Check sheet for the modelled part. Datum: model origin and axes. Units: mm. Face numbers are marked on the shaded views. A direction names the side the tool comes from. Round coordinates to 2 decimals unless told otherwise and drop trailing zeros. Loops run counter-clockwise (first coordinate to the right, second up) from the corner with the lowest first, then second, coordinate; pieces in that order, holes last. Notation, with made-up numbers: (-37, 38.5) - (-4, 38.5) arc R36 ccw to (-4, 74.5) - close; hole circle Ø1 at (-18, 37.25). An arc over 180 degrees is marked (long way). Put each result on its own line as item: value. Start each with the question number.
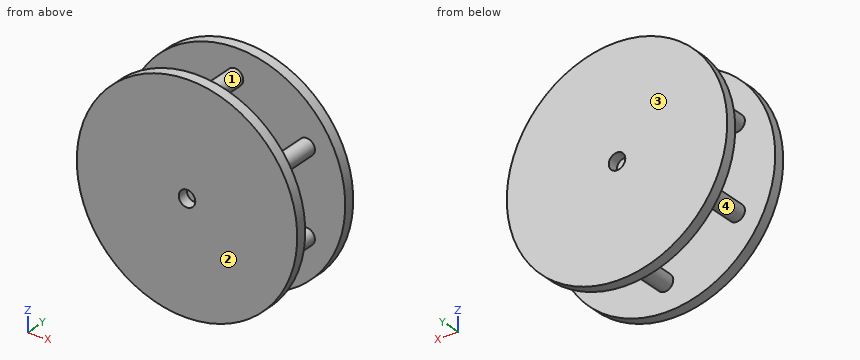
```python
from build123d import *

# Parameters (mm, degrees)
SKETCH1_R           = 50.789558068
BOSS_EXTRUDE1_DEPTH = 5.08
SKETCH3_R           = 3.813733887
BOSS_EXTRUDE2_DEPTH = 25.4
CIRPATTERN1_COUNT   = 6
SKETCH4_R           = 50.789558068
BOSS_EXTRUDE3_DEPTH = 5.08
SKETCH6_R           = 3.81
CUT_EXTRUDE1_DEPTH  = 81.147813554


with BuildPart() as part:
    # Sketch1 → Boss-Extrude1 (new body)
    with BuildSketch(Plane(origin=(0, 0, 0), x_dir=(1, 0, 0), z_dir=(0, 1, 0))):
        with Locations(Location((0, 0, 0), (0, 0, 270))):
            Circle(SKETCH1_R)
    extrude(amount=BOSS_EXTRUDE1_DEPTH)

    # Sketch3 → Boss-Extrude2 (add)
    with BuildSketch(Plane(origin=(0, 5.08, 0), x_dir=(1, 0, 0), z_dir=(0, 1, 0))):
        with Locations(Location((0, 38.1, 0), (0, 0, 270))):
            Circle(SKETCH3_R)
    boss_extrude2 = extrude(amount=BOSS_EXTRUDE2_DEPTH)

    # CirPattern1: Boss-Extrude2 ×6 about axis
    cirpattern1_axis = Axis((0, 0, 0), (0, 1, 0))
    for i in range(1, CIRPATTERN1_COUNT):
        add(boss_extrude2.rotate(cirpattern1_axis, i * 360 / CIRPATTERN1_COUNT))

    # Sketch4 → Boss-Extrude3 (add)
    with BuildSketch(Plane(origin=(0, 30.48, 0), x_dir=(1, 0, 0), z_dir=(0, 1, 0))):
        with Locations(Location((0, 0, 0), (0, 0, 270))):
            Circle(SKETCH4_R)
    extrude(amount=BOSS_EXTRUDE3_DEPTH)

    # Sketch6 → Cut-Extrude1 (cut, through all)
    with BuildSketch(Plane(origin=(0, 35.56, 0), x_dir=(1, 0, 0), z_dir=(0, 1, 0))):
        with Locations(Location((0, 0, 0), (0, 0, 270))):
            Circle(SKETCH6_R)
    extrude(amount=-CUT_EXTRUDE1_DEPTH, mode=Mode.SUBTRACT)


solid = part.part
```
Q1. Depth check by flat-ended pin: pin 1 Ø10 at (y, z) = (13, -27) entering from -X; pin 2 Ø10 at (x, y) = (-3, 25) entering from -Z; pin 3 Ø4 at (x, y) = (-4, 23) entering from +Z; pin 4 Ø1 at (x, y) = (5, 26.5) entering from -Z. Enter the tip coordinate at first touch or a pass-through.
Q2. Cross-section at A-A on x = 0. Enter the section's corners in (y, z).
Q3. Cross-section at C-C on y = 23. Enter the section's corners in (x, z), and give its area (3 significant figures).
Q4. Cross-section at D-D on z = 19.05. Enter the section's corners in (x, y).
Q5. Cross-section at B-B on z = 0. Enter the section's corners in (x, y).
Q6. Draft check along Z on the marked faces 3 and 4. Enter one of: +Z half, -Z half, draft (parallel to the pull), parting line (faces both ways), or undercut.
Q7. Material ranges on line 1 (Y direction, x = -40, z = 2.5); line 2 (X direction, y = 32.45, z = 0); line 3 (Z direction, x = -2.5, y = 19.5), recorded low to high. Write a range as from..to.
Q8. Set-up check for the marked faces 1 and 2: record each of +Z, -Z, +X, -X, +Y, -Y from which the full face is reachable in a straight line by a thin tool's end or side.
Answer list:
1. pin 1: stops at x = -35.41
1. pin 2: stops at z = -41.91
1. pin 3: stops at z = 41.35
1. pin 4: passes through
2. outline: (0, -50.79) - (5.08, -50.79) - (5.08, -41.91) - (30.48, -41.91) - (30.48, -50.79) - (35.56, -50.79) - (35.56, -3.81) - (30.48, -3.81) - (30.48, -34.29) - (5.08, -34.29) - (5.08, -3.81) - (0, -3.81) - close; (0, 3.81) - (5.08, 3.81) - (5.08, 34.29) - (30.48, 34.29) - (30.48, 3.81) - (35.56, 3.81) - (35.56, 50.79) - (30.48, 50.79) - (30.48, 41.91) - (5.08, 41.91) - (5.08, 50.79) - (0, 50.79) - close
3. outline: circle Ø7.63 at (-33, -19.05); circle Ø7.63 at (-33, 19.05); circle Ø7.63 at (0, -38.1); circle Ø7.63 at (0, 38.1); circle Ø7.63 at (33, -19.05); circle Ø7.63 at (33, 19.05)
3. area: 274 mm2
4. outline: (-47.08, 0) - (47.08, 0) - (47.08, 5.08) - (36.81, 5.08) - (36.81, 30.48) - (47.08, 30.48) - (47.08, 35.56) - (-47.08, 35.56) - (-47.08, 30.48) - (-36.81, 30.48) - (-36.81, 5.08) - (-47.08, 5.08) - close; hole (-29.18, 5.08) - (29.18, 5.08) - (29.18, 30.48) - (-29.18, 30.48) - close
5. outline: (-50.79, 0) - (-3.81, 0) - (-3.81, 5.08) - (-50.79, 5.08) - close; (-50.79, 30.48) - (-3.81, 30.48) - (-3.81, 35.56) - (-50.79, 35.56) - close; (3.81, 0) - (50.79, 0) - (50.79, 5.08) - (3.81, 5.08) - close; (3.81, 30.48) - (50.79, 30.48) - (50.79, 35.56) - (3.81, 35.56) - close
6. face 3: draft
6. face 4: undercut
7. line 1: y = 0..5.08, 30.48..35.56
7. line 2: x = -50.79..-3.81, 3.81..50.79
7. line 3: z = -40.98..-35.22, 35.22..40.98
8. face 1: none
8. face 2: +Z, -Z, +X, -X, -Y
